The listing builds one solid part. Answer for the finished solid, in the listing's coordinates (mm). Face numbers are marked on the shaded views. A direction names the side the tool comes from. Round coordinates to 2 decimals unless told otherwise and drop trailing zeros. Order: outer loops, then holes, each group sorted by start corner. A loop starts at its lowest first (then second) coordinate and runs counter-clockwise, first axis right, second up. Notation, with made-up numbers: (84, 0.5) - (133, 0.5) arc R8 cw to (133, 13.5) - close; hole circle Ø10 at (-28, -39). An arc over 180 degrees is marked (long way). One line per item, written item: value. Start each with the question number.
1. Section A-A, the plane y = -2.25 is taken. Give the vertices of the cut face in (x, z).
2. Section D-D, the plane x = -5 is taken. Give the vertices of the cut face in (y, z) (3 decimals).
3. Section B-B, the plane z = 3.25 is taken. Give the vertices of the cut face in (x, y).
4. A tool of negligible diameter and unlimited length cuts with its end or side. For the marked faces 1, 2, 3 and 4, from which of +Z, -Z, +X, -X, +Y, -Y can it reach the whole face along a straight path? Write none if from no direction.
5. For a pull along X with two mould halves and no side action, classify the marked faces 5, 6 and 7 as released by +X, released by -X, zero draft, split by the parting line, or undercut.
6. Straight lines are drawn through the part: line 1 (X direction, y = 10.8, z = 0); line 2 (X direction, y = 3.25, z = 0); line 3 (Y direction, x = 4, z = -1). For each, find the intervals that lie inside material, in ascending order.
7. Flat-ended cylindrical pins translate along their axes: P1, Ø0.6, axis at y = -1, z = -0.5, coming from the +X side; P2, Ø0.8, axis at x = 0, y = -2.5, coming from the +Z side; P3, Ø2, axis at x = -6, y = 3.5, coming from the +Z side. Find the tip coordinate at first contact, or state that the pin passes through.
8. Section C-C, the plane y = 2 is taken. Give the vertices of the cut face in (x, z).
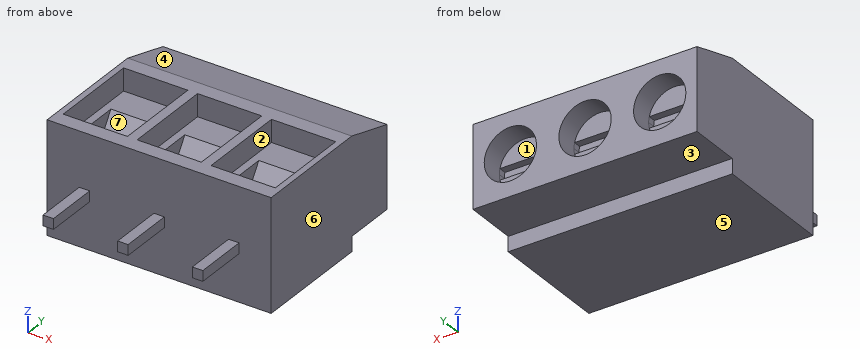
from build123d import *
from OCP.BRepFilletAPI import BRepFilletAPI_MakeChamfer

# Parameters (mm, degrees)
SKETCH1_W           = 15
SKETCH1_H           = 7.5
BOSS_EXTRUDE1_DEPTH = 11.5
SKETCH2_W           = 1
SKETCH2_H           = 3.5
CUT_EXTRUDE1_DEPTH  = 20.269470673
CUT_EXTRUDE2_DEPTH  = 20.269470673
SKETCH4_R           = 1.75
CUT_EXTRUDE3_DEPTH  = 1.5
SKETCH5_W           = 3.418698582
SKETCH5_H           = 0.75
CUT_EXTRUDE4_DEPTH  = 0.5
SKETCH6_W           = 4.3
SKETCH6_H           = 6
CUT_EXTRUDE5_DEPTH  = 1.5
SKETCH7_W           = 3.3
SKETCH7_H           = 1.5
CUT_EXTRUDE6_DEPTH  = 5
CHAMFER1_SIZE       = 2
CHAMFER1_SIZE2      = 3
SKETCH8_W           = 0.7
SKETCH8_H           = 0.7
BOSS_EXTRUDE2_DEPTH = 3.6


with BuildPart() as part:
    # Sketch1 → Boss-Extrude1 (new body)
    with BuildSketch(Plane(origin=(0, 0, 0), x_dir=(1, 0, 0), z_dir=(0, 1, 0))):
        Rectangle(SKETCH1_W, SKETCH1_H)
    extrude(amount=BOSS_EXTRUDE1_DEPTH)

    # Sketch2 → Cut-Extrude1 (cut, through all)
    with BuildSketch(Plane.ZY.offset(7.5)):
        with Locations((-3.25, 9.75)):
            Rectangle(SKETCH2_W, SKETCH2_H)
    extrude(amount=-CUT_EXTRUDE1_DEPTH, mode=Mode.SUBTRACT)

    # Sketch3 → Cut-Extrude2 (cut, through all)
    with BuildSketch(Plane.ZY.offset(7.5)):
        Polygon((3.75, 8), (2.75, 11.5), (3.75, 11.5), align=None)
    extrude(amount=-CUT_EXTRUDE2_DEPTH, mode=Mode.SUBTRACT)

    # Sketch4 → Cut-Extrude3 (cut)
    with BuildSketch(Plane(origin=(0, 11.5, 0), x_dir=(1, 0, 0), z_dir=(0, 1, 0))):
        with Locations(Location((-5, 0, 0), (0, 0, 270))):
            Circle(SKETCH4_R)
        with Locations(Location((0, 0, 0), (0, 0, 270))):
            Circle(SKETCH4_R)
        with Locations(Location((5, 0, 0), (0, 0, 270))):
            Circle(SKETCH4_R)
    extrude(amount=-CUT_EXTRUDE3_DEPTH, mode=Mode.SUBTRACT)

    # Sketch5 → Cut-Extrude4 (cut)
    with BuildSketch(Plane(origin=(0, 10, 0), x_dir=(1, 0, 0), z_dir=(0, 1, 0))):
        with Locations((-5, 0)):
            Rectangle(SKETCH5_W, SKETCH5_H)
        with BuildLine():
            Line((-6.709349291, -0.375), (-6.709349291, 0.375))
            ThreePointArc((-6.709349291, 0.375), (-6.75, 0), (-6.709349291, -0.375))
        make_face()
        with BuildLine():
            ThreePointArc((-3.25, 0), (-3.260192358, 0.188598436), (-3.290650709, 0.375))
            Line((-3.290650709, 0.375), (-3.290650709, -0.375))
            ThreePointArc((-3.290650709, -0.375), (-3.260192358, -0.188598436), (-3.25, 0))
        make_face()
        Rectangle(SKETCH5_W, SKETCH5_H)
        with BuildLine():
            ThreePointArc((1.75, 0), (1.739807642, 0.188598436), (1.709349291, 0.375))
            Line((1.709349291, 0.375), (1.709349291, -0.375))
            ThreePointArc((1.709349291, -0.375), (1.739807642, -0.188598436), (1.75, 0))
        make_face()
        with Locations((5, 0)):
            Rectangle(SKETCH5_W, SKETCH5_H)
        with BuildLine():
            ThreePointArc((6.75, 0), (6.739807642, 0.188598436), (6.709349291, 0.375))
            Line((6.709349291, 0.375), (6.709349291, -0.375))
            ThreePointArc((6.709349291, -0.375), (6.739807642, -0.188598436), (6.75, 0))
        make_face()
        with BuildLine():
            Line((3.290650709, -0.375), (3.290650709, 0.375))
            ThreePointArc((3.290650709, 0.375), (3.25, 0), (3.290650709, -0.375))
        make_face()
        with BuildLine():
            Line((-1.709349291, -0.375), (-1.709349291, 0.375))
            ThreePointArc((-1.709349291, 0.375), (-1.75, 0), (-1.709349291, -0.375))
        make_face()
    extrude(amount=-CUT_EXTRUDE4_DEPTH, mode=Mode.SUBTRACT)

    # Sketch6 → Cut-Extrude5 (cut)
    with BuildSketch(Plane.XY.offset(3.75)):
        with Locations((-4.95, 4)):
            Rectangle(SKETCH6_W, SKETCH6_H)
        with Locations((0, 4)):
            Rectangle(SKETCH6_W, SKETCH6_H)
        with Locations((4.95, 4)):
            Rectangle(SKETCH6_W, SKETCH6_H)
    extrude(amount=-CUT_EXTRUDE5_DEPTH, mode=Mode.SUBTRACT)

    # Sketch7 → Cut-Extrude6 (cut)
    with BuildSketch(Plane.XY.offset(2.25)):
        with Locations((-4.95, 2.25)):
            Rectangle(SKETCH7_W, SKETCH7_H)
        with Locations((0, 2.25)):
            Rectangle(SKETCH7_W, SKETCH7_H)
        with Locations((4.95, 2.25)):
            Rectangle(SKETCH7_W, SKETCH7_H)
    extrude(amount=-CUT_EXTRUDE6_DEPTH, mode=Mode.SUBTRACT)

    # Chamfer1: one chamfer whose edges measure the first distance from different faces: ONE call of the kernel's chamfer builder (chamfer() names one face for all edges)
    chamfer1_edges_1 = [part.edges().sort_by_distance(p)[0] for p in [
        (-4.95, 3, 2.25),
    ]]
    chamfer1_side_1 = [part.faces().sort_by_distance(p)[0] for p in [
        (-4.95, 4.415467626, 2.25),
    ]]
    chamfer1_edges_2 = [part.edges().sort_by_distance(p)[0] for p in [
        (0, 3, 2.25),
    ]]
    chamfer1_side_2 = [part.faces().sort_by_distance(p)[0] for p in [
        (0, 4.415467626, 2.25),
    ]]
    chamfer1_edges_3 = [part.edges().sort_by_distance(p)[0] for p in [
        (4.95, 3, 2.25),
    ]]
    chamfer1_side_3 = [part.faces().sort_by_distance(p)[0] for p in [
        (4.95, 4.415467626, 2.25),
    ]]
    chamfer1 = BRepFilletAPI_MakeChamfer(part.part.solid().wrapped)
    for e in chamfer1_edges_1:
        chamfer1.Add(CHAMFER1_SIZE, CHAMFER1_SIZE2, e.wrapped, chamfer1_side_1[0].wrapped)  # the first distance lies on this face
    for e in chamfer1_edges_2:
        chamfer1.Add(CHAMFER1_SIZE, CHAMFER1_SIZE2, e.wrapped, chamfer1_side_2[0].wrapped)  # the first distance lies on this face
    for e in chamfer1_edges_3:
        chamfer1.Add(CHAMFER1_SIZE, CHAMFER1_SIZE2, e.wrapped, chamfer1_side_3[0].wrapped)  # the first distance lies on this face
    add(Compound.cast(chamfer1.Shape()), mode=Mode.REPLACE)

    # Sketch8 → Boss-Extrude2 (add)
    with BuildSketch(Plane.XZ):
        with Locations((-5, -0.25)):
            Rectangle(SKETCH8_W, SKETCH8_H)
        with Locations((0, -0.25)):
            Rectangle(SKETCH8_W, SKETCH8_H)
        with Locations((5, -0.25)):
            Rectangle(SKETCH8_W, SKETCH8_H)
    extrude(amount=BOSS_EXTRUDE2_DEPTH)


solid = part.part
Answer list:
1. outline: (-5.35, -0.6) - (-4.65, -0.6) - (-4.65, 0.1) - (-5.35, 0.1) - close; (-0.35, -0.6) - (0.35, -0.6) - (0.35, 0.1) - (-0.35, 0.1) - close; (4.65, -0.6) - (5.35, -0.6) - (5.35, 0.1) - (4.65, 0.1) - close
2. outline: (-3.6, -0.6) - (0, -0.6) - (0, -3.75) - (8, -3.75) - (8, -2.75) - (11.5, -2.75) - (11.5, -1.75) - (10, -1.75) - (10, -0.375) - (9.5, -0.375) - (9.5, 0.375) - (10, 0.375) - (10, 1.75) - (11.5, 1.75) - (11.5, 2.75) - (8, 3.75) - (7, 3.75) - (7, 2.25) - (5, 2.25) - (3, -0.75) - (3, -2.75) - (1.5, -2.75) - (1.5, 2.25) - (1, 2.25) - (1, 3.75) - (0, 3.75) - (0, 0.1) - (-3.6, 0.1) - close
3. outline: (-7.5, 0) - (7.5, 0) - (7.5, 9.75) - (-7.5, 9.75) - close; hole (-7.1, 1) - (-2.8, 1) - (-2.8, 7) - (-7.1, 7) - close; hole (-2.15, 1) - (2.15, 1) - (2.15, 7) - (-2.15, 7) - close; hole (2.8, 1) - (7.1, 1) - (7.1, 7) - (2.8, 7) - close
4. face 1: +Y
4. face 2: +Z
4. face 3: -Z, +X, -X, +Y
4. face 4: +Z, +X, -X, +Y
5. face 5: zero draft
5. face 6: released by +X
5. face 7: undercut
6. line 1: x = -7.5 to -6.75, -3.25 to -1.75, 1.75 to 3.25, 6.75 to 7.5
6. line 2: x = -7.5 to -6.6, -3.3 to -1.65, 1.65 to 3.3, 6.6 to 7.5
6. line 3: y = 0 to 1.5, 3 to 10
7. P1: stops at x = 5.35
7. P2: stops at z = 0.1
7. P3: stops at z = 2.25
8. outline: (-7.5, -3.75) - (7.5, -3.75) - (7.5, 3.75) - (7.1, 3.75) - (7.1, 2.25) - (6.6, 2.25) - (6.6, -2.75) - (3.3, -2.75) - (3.3, 2.25) - (2.8, 2.25) - (2.8, 3.75) - (2.15, 3.75) - (2.15, 2.25) - (1.65, 2.25) - (1.65, -2.75) - (-1.65, -2.75) - (-1.65, 2.25) - (-2.15, 2.25) - (-2.15, 3.75) - (-2.8, 3.75) - (-2.8, 2.25) - (-3.3, 2.25) - (-3.3, -2.75) - (-6.6, -2.75) - (-6.6, 2.25) - (-7.1, 2.25) - (-7.1, 3.75) - (-7.5, 3.75) - close
